Source: three-view drawing plus pictorial views. Frame: mm from the lowest corner of the part. Give positions to 0.01 mm unless a question says otherwise; leave off trailing zeros. Write each loop counter-clockwise with the first axis right and the second up, starting at its lowest first coordinate (ties: lowest second). Pieces come first, ordered by that corner, then holes.
Q1. Cut plane C-C on x = 134. Return the cut outline in (y, z).
Q2. Cut plane A-A on z = 1.55. Return the cut outline in (x, y).
Q3. Cut plane B-B on y = 29. Return the cut outline in (x, z), plus the area to 3 significant figures.
Q4. Pin query (flat end, axial travel): pin 1 (1.3 mm diameter, centred on x = 24.5, z = 1.5, fed in from -Y); pin 2 (1.3 mm diameter, centred on y = 89.5, z = 1, fed in from +X); pin 3 (0.8 mm diameter, centred on y = 64, z = 1, fed in from -X). Return the tip coordinate at first contact, or that it passes through.
Q5. Line query: L1, parallel to Y at x = 66, z = 2; L2, parallel to X at y = 24.5, z = 1.9. Output: solid intervals per line, ascending.
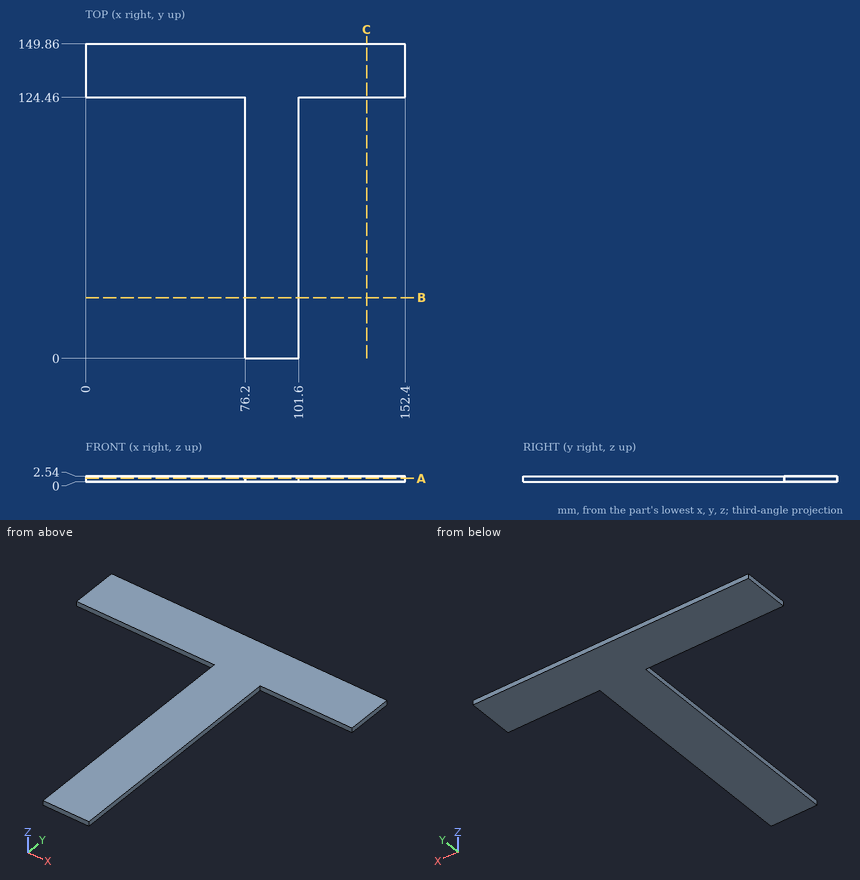
Data:
1. outline: (124.46, 0) - (149.86, 0) - (149.86, 2.54) - (124.46, 2.54) - close
2. outline: (0, 124.46) - (76.2, 124.46) - (76.2, 0) - (101.6, 0) - (101.6, 124.46) - (152.4, 124.46) - (152.4, 149.86) - (0, 149.86) - close
3. outline: (76.2, 0) - (101.6, 0) - (101.6, 2.54) - (76.2, 2.54) - close
3. area: 64.5 mm2
4. pin 1: stops at y = 124.46
4. pin 2: stops at x = 101.6
4. pin 3: stops at x = 76.2
5. L1: y = 124.46 to 149.86
5. L2: x = 76.2 to 101.6
